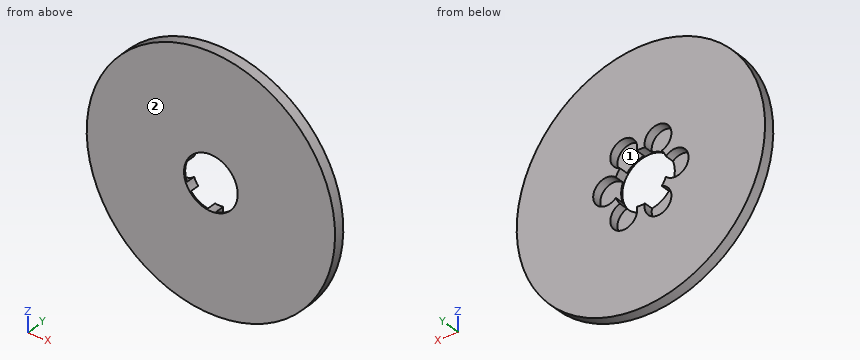
```python
from build123d import *

# Parameters (mm, degrees)
SKETCH1_R           = 92.5
BOSS_EXTRUDE1_DEPTH = 8
SKETCH2_R           = 20
CUT_EXTRUDE1_DEPTH  = 132.059146953
SKETCH3_R           = 10
CUT_EXTRUDE2_DEPTH  = 6.885448
CIRPATTERN1_START   = 1.114552302
CIRPATTERN1_DEPTH   = 6.885447698


# Read off the part's stored shape, not the designer's step: CirPattern1
with BuildPart() as part:
    # Sketch1 → Boss-Extrude1 (new body)
    with BuildSketch(Plane(origin=(0, 0, 0), x_dir=(1, 0, 0), z_dir=(0, 1, 0))):
        with Locations(Location((0, 0, 0), (0, 0, 270))):
            Circle(SKETCH1_R)
    extrude(amount=BOSS_EXTRUDE1_DEPTH)

    # Sketch2 → Cut-Extrude1 (cut, through all)
    with BuildSketch(Plane(origin=(0, 0, 0), x_dir=(1, 0, 0), z_dir=(0, 1, 0))):
        with Locations(Location((0, 0, 0), (0, 0, 270))):
            Circle(SKETCH2_R)
    extrude(amount=CUT_EXTRUDE1_DEPTH, mode=Mode.SUBTRACT)

    # Sketch3 → Cut-Extrude2 (cut)
    with BuildSketch(Plane(origin=(0, 8, 0), x_dir=(1, 0, 0), z_dir=(0, 1, 0))):
        with Locations((-25.516109786, 0)):
            Circle(SKETCH3_R)
    extrude(amount=-CUT_EXTRUDE2_DEPTH, mode=Mode.SUBTRACT)

    # CirPattern1 outline → CirPattern1 (cut)
    with BuildSketch(Plane(origin=(0, 0, 0), x_dir=(1, 0, 0), z_dir=(0, 1, 0)).offset(CIRPATTERN1_START)):
        with BuildLine():
            ThreePointArc((-3.033028496, -19.768680739), (-10, -17.320508076), (-15.603665471, -12.511020097))
            ThreePointArc((-15.603665471, -12.511020097), (-17.758054893, -30.757853318), (-3.033028496, -19.768680739))
        make_face()
        with BuildLine():
            ThreePointArc((-3.033028496, 19.768680739), (-17.758054893, 30.757853318), (-15.603665471, 12.511020097))
            ThreePointArc((-15.603665471, 12.511020097), (-10, 17.320508076), (-3.033028496, 19.768680739))
        make_face()
        with BuildLine():
            ThreePointArc((15.603665471, -12.511020097), (10, -17.320508076), (3.033028496, -19.768680739))
            ThreePointArc((3.033028496, -19.768680739), (17.758054893, -30.757853318), (15.603665471, -12.511020097))
        make_face()
        with BuildLine():
            ThreePointArc((15.603665471, 12.511020097), (17.758054893, 30.757853318), (3.033028496, 19.768680739))
            ThreePointArc((3.033028496, 19.768680739), (10, 17.320508076), (15.603665471, 12.511020097))
        make_face()
        with BuildLine():
            ThreePointArc((18.636693967, 7.257660642), (20, 0), (18.636693967, -7.257660642))
            ThreePointArc((18.636693967, -7.257660642), (35.516109786, 0), (18.636693967, 7.257660642))
        make_face()
    extrude(amount=CIRPATTERN1_DEPTH, mode=Mode.SUBTRACT)


solid = part.part
```
Work out the finished part from the listing and answer in its coordinate system (mm). Face numbers are marked on the shaded views. Give positions to 0.01 mm unless a question says otherwise; leave off trailing zeros. Write each loop counter-clockwise with the first axis right and the second up, starting at its lowest first coordinate (ties: lowest second). Pieces come first, ordered by that corner, then holes. Notation, with made-up numbers: (-3.5, 30.25) -> (33.5, 30.25) arc R12 ccw to (33.5, 43.25) -> close; hole circle Ø6 at (83, 54). An arc over 180 degrees is marked (long way). Write item = value, one per line.
Q1. Consider line 1 along X through (y, z) = (4.75, 0); line 2 along X through (y, z) = (4, 28); line 3 along Z through (x, y) = (-4.5, 5.5). Determine where each line is inside the solid, lowest interval first.
Computed values:
line_1 = -92.5 to -35.52, 35.52 to 92.5
line_2 = -88.16 to -20.83, -4.69 to 4.69, 20.83 to 88.16
line_3 = -92.39 to -27.74, 27.74 to 92.39
Q2. For a pull along Z with two mould halves and no side action, classify the marked faces 1 and 2 as pulls with the +Z half, pulls with the -Z half, needs draft (parallel to the pull), parting line crosses it, or undercut.
Computed values:
face_1 = undercut
face_2 = needs draft
Q3. Section C-C on y = 5.75 is taken. Determine the outline of the cut face in (x, z).
Computed values:
outline = circle Ø185 at (0, 0); hole (-18.64, -7.26) arc R20 ccw to (-15.6, -12.51) arc R10 ccw (long way) to (-3.03, -19.77) arc R20 ccw to (3.03, -19.77) arc R10 ccw (long way) to (15.6, -12.51) arc R20 ccw to (18.64, -7.26) arc R10 ccw (long way) to (18.64, 7.26) arc R20 ccw to (15.6, 12.51) arc R10 ccw (long way) to (3.03, 19.77) arc R20 ccw to (-3.03, 19.77) arc R10 ccw (long way) to (-15.6, 12.51) arc R20 ccw to (-18.64, 7.26) arc R10 ccw (long way) to start
Q4. Section A-A on z = 0 is taken. Determine the outline of the cut face in (x, y).
Computed values:
outline = (-92.5, 0) -> (-20, 0) -> (-20, 1.11) -> (-35.52, 1.11) -> (-35.52, 8) -> (-92.5, 8) -> close; (20, 0) -> (92.5, 0) -> (92.5, 8) -> (35.52, 8) -> (35.52, 1.11) -> (20, 1.11) -> close
Q5. Section B-B on x = 0 is taken. Determine the outline of the cut face in (y, z).
Computed values:
outline = (0, -92.5) -> (8, -92.5) -> (8, -20) -> (0, -20) -> close; (0, 20) -> (8, 20) -> (8, 92.5) -> (0, 92.5) -> close
Q6. Flat-ended cylindrical pins translate along their axes: pin 1 Ø1 at (y, z) = (3.5, 73.5) entering from +X; pin 2 Ø18 at (x, z) = (-12.76, 22.1) entering from +Y; pin 3 Ø4 at (y, z) = (5.5, -35.5) entering from -X. Find the tip coordinate at first contact, or state that the pin passes through.
Computed values:
pin_1 = 56.81
pin_2 = 1.11
pin_3 = -86.22
Q7. Section D-D on x = -33 is taken. Determine the outline of the cut face in (y, z), and give its area (3 significant figures).
Computed values:
outline = (0, -86.41) -> (8, -86.41) -> (8, -6.63) -> (1.11, -6.63) -> (1.11, 6.63) -> (8, 6.63) -> (8, 86.41) -> (0, 86.41) -> close
area = 1,290 mm^2
